The listing builds one solid part. Answer for the finished solid, in the listing's coordinates (mm). A direction names the side the tool comes from. Round coordinates to 2 decimals unless told otherwise and drop trailing zeros. Write each loop counter-clockwise with the first axis right and the second up, starting at its lowest first coordinate (ties: lowest second). Pieces come first, ordered by that corner, then holes. Notation, with made-up numbers: (1, -2.5) - (46, -2.5) arc R20 ccw to (46, 6.5) - close; hole circle Ø8 at (53, 42). An arc over 180 degrees is marked (long way). Return JSON: item names as keys, results as strings. Group by question number.
(1) Section D-D, the plane x = 0 is taken. Write down the section's boundary in (y, z).
(2) Find the intervals of material crossed by line 1 along X through (y, z) = (4.5, 37); line 2 along Z through (x, y) = (-19.75, 0); line 3 along X through (y, z) = (3.75, 7.5), in increasing order. Write a range as [from, to].
(3) Section C-C, the plane y = 0 is taken. Write down the section's boundary in (x, z).
(4) Which of the six approach directions +Z, -Z, +X, -X, +Y, -Y give full straight-line access (tool end or side, diameter ignored) to faces 5 (the flat face through (6, 8.167, 17)), 6 (the flat face through (-25.4, 0, 27)), 7 (the flat face through (25.4, 0, 27)), 8 (the flat face through (-9.828, 0, 35))?
(5) Section B-B, the plane z = 19.5 is taken. Write down the section's boundary in (x, y), then the cut area to 3 significant figures.
(6) Section A-A, the plane x = 46 is taken. Write down the section's boundary in (y, z), then the cut area to 3 significant figures.
(7) Each of these flat-tipped pins is pushed along its axis until it touches: pin 1 (10.5 mm diameter, centred on y = 0, z = 41.38, fed in from +X); pin 2 (5 mm diameter, centred on x = 38.5, y = 1, fed in from -Z); pin 3 (5 mm diameter, centred on y = -4, z = 37, fed in from -X); pin 4 (4 mm diameter, centred on x = 19.5, z = 44, fed in from +Y). Where does it stop, or does it pass through?
(8) Determine the mould class of faces 1 (the cylindrical face through (17.86, 2.4, 45.14)), 2 (the cylindrical face through (39.755, 0.316, 6.439)), 3 (the cylindrical face through (-17.51, 0.18, 49.55)), 4 (the flat face through (6, -8.167, 18)) for opening direction Y: +Y half, -Y half, draft (parallel to the pull), parting line (faces both ways), or undercut.
```python
from build123d import *

# Parameters (mm, degrees)
F1_DEPTH = 12.7
F2_R     = 7.177953
F2_R_2   = 5.665959
F3_DEPTH = 25.4
F5_DEPTH = 25.4
F6_R     = 4.457647
F7_DEPTH = 63.5
F9_DEPTH = 38.1


with BuildPart() as f1:
    # F0 (on Top) → F1 (new body)
    with BuildSketch(Plane.XY):
        with BuildLine():
            ThreePointArc((44.840731, -14.530204), (61.605395, 0), (44.840731, 14.530204))
            Line((44.840731, 14.530204), (-46.926282, 14.530204))
            Line((-46.926282, 14.530204), (-46.926282, 14.414141))
            ThreePointArc((-46.926282, 14.414141), (-61.340423, 0), (-46.926282, -14.414141))
            Line((-46.926282, -14.414141), (-46.926282, -14.530204))
            Line((-46.926282, -14.530204), (44.840731, -14.530204))
        make_face()
    extrude(amount=F1_DEPTH)

    # F2 (on face) → F3 (cut)
    with BuildSketch(Plane.XY.offset(12.7)):
        with Locations((46.926282, 0)):
            Circle(F2_R)
        with Locations((-46.926282, 0)):
            Circle(F2_R_2)
    extrude(amount=-F3_DEPTH, mode=Mode.SUBTRACT)

    # F4 (on Right) → F5 (join, symmetric)
    with BuildSketch(Plane.YZ):
        with BuildLine():
            Line((-8.16711, 12.592246), (8.16711, 12.592246))
            Line((8.16711, 12.592246), (8.16711, 41.384771))
            ThreePointArc((8.16711, 41.384771), (0, 49.551881), (-8.16711, 41.384771))
            Line((-8.16711, 41.384771), (-8.16711, 12.592246))
        make_face()
    extrude(amount=F5_DEPTH, both=True)

    # F6 (on face) → F7 (cut, symmetric)
    with BuildSketch(Plane.YZ.offset(25.4)):
        with Locations((0, 41.384771)):
            Circle(F6_R)
    extrude(amount=F7_DEPTH, both=True, mode=Mode.SUBTRACT)

    # F8 (on Front) → F9 (cut, symmetric)
    with BuildSketch(Plane.XZ):
        with BuildLine():
            Line((10.105069, 50.244011), (-9.828218, 50.244011))
            Line((-9.828218, 50.244011), (-9.828218, 29.614518))
            ThreePointArc((-9.828218, 29.614518), (-1.182707, 17.229743), (10.105069, 27.265361))
            Line((10.105069, 27.265361), (10.105069, 50.244011))
        make_face()
    extrude(amount=F9_DEPTH, both=True, mode=Mode.SUBTRACT)


solid = f1.part
```
Working result:
{
 "1": {"outline": "(-14.53, 0) - (14.53, 0) - (14.53, 12.7) - (8.17, 12.7) - (8.17, 17.16) - (-8.17, 17.16) - (-8.17, 12.7) - (-14.53, 12.7) - close"},
 "2": {"line 1": "x = [-25.4, -9.83], [10.11, 25.4]", "line 2": "z = [0, 36.93], [45.84, 49.55]", "line 3": "x = [-60.84, -51.17], [-42.68, 40.81], [53.05, 61.12]"},
 "3": {"outline": "(-61.34, 0) - (-52.59, 0) - (-52.59, 12.7) - (-61.34, 12.7) - close; (-41.26, 0) - (39.75, 0) - (39.75, 12.7) - (25.4, 12.7) - (25.4, 36.93) - (10.11, 36.93) - (10.11, 27.27) arc R10.11 cw (long way) to (-9.83, 29.61) - (-9.83, 36.93) - (-25.4, 36.93) - (-25.4, 12.7) - (-41.26, 12.7) - close; (-25.4, 45.84) - (-9.83, 45.84) - (-9.83, 49.55) - (-25.4, 49.55) - close; (10.11, 45.84) - (25.4, 45.84) - (25.4, 49.55) - (10.11, 49.55) - close; (54.1, 0) - (61.61, 0) - (61.61, 12.7) - (54.1, 12.7) - close"},
 "4": {"face 5": "+Z, +X, -X, +Y", "face 6": "+Z, -X, +Y, -Y", "face 7": "+Z, +X, +Y, -Y", "face 8": "+Z, +Y, -Y"},
 "5": {"outline": "(-25.4, -8.17) - (-6.47, -8.17) - (-6.47, 8.17) - (-25.4, 8.17) - close; (6.47, -8.17) - (25.4, -8.17) - (25.4, 8.17) - (6.47, 8.17) - close", "area": "619 mm^2"},
 "6": {"outline": "(-14.65, 0) - (-7.12, 0) - (-7.12, 12.7) - (-14.65, 12.7) - close; (7.12, 0) - (14.65, 0) - (14.65, 12.7) - (7.12, 12.7) - close", "area": "191 mm^2"},
 "7": {"pin 1": "stops at x = 25.4", "pin 2": "stops at z = 0", "pin 3": "stops at x = -25.4", "pin 4": "stops at y = 8.14"},
 "8": {"face 1": "undercut", "face 2": "undercut", "face 3": "parting line", "face 4": "-Y half"}
}
